The model under review builds one solid part; all positions refer to its coordinate system, in mm. Face numbers are marked on the shaded views. A direction names the side the tool comes from. Round coordinates to 2 decimals unless told otherwise and drop trailing zeros. Write each loop counter-clockwise with the first axis right and the second up, starting at its lowest first coordinate (ties: lowest second). Pieces come first, ordered by that corner, then holes. Notation, with made-up numbers: (-16.5, 72) -> (9.5, 72) arc R22 ccw to (9.5, 109) -> close; hole circle Ø9 at (-32.5, -24.75). An arc over 180 degrees is marked (long way). Answer in a Markdown table with one row per item. Add a question column.
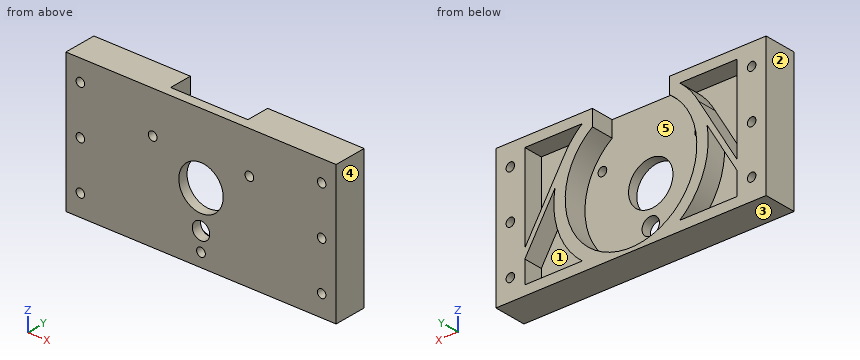
```python
from build123d import *

# Parameters (mm, degrees)
SKETCH1_W           = 140
SKETCH1_H           = 72
BOSS_EXTRUDE1_DEPTH = 17
SKETCH2_R           = 34.1
CUT_EXTRUDE1_DEPTH  = 12
SKETCH3_W           = 40
SKETCH3_H           = 24
CUT_EXTRUDE2_DEPTH  = 10
SKETCH4_R           = 2.2
CUT_EXTRUDE3_DEPTH  = 81.529497701
SKETCH5_R           = 2.25
SKETCH5_R_2         = 4.5
CUT_EXTRUDE4_DEPTH  = 80.62411695
CUT_EXTRUDE5_DEPTH  = 10
SKETCH7_R           = 11.5
CUT_EXTRUDE6_DEPTH  = 10


with BuildPart() as part:
    # Sketch1 → Boss-Extrude1 (new body)
    with BuildSketch(Plane(origin=(0, 0, 0), x_dir=(1, 0, 0), z_dir=(0, 1, 0))):
        Rectangle(SKETCH1_W, SKETCH1_H)
    extrude(amount=BOSS_EXTRUDE1_DEPTH)

    # Sketch2 → Cut-Extrude1 (cut)
    with BuildSketch(Plane(origin=(0, 17, 0), x_dir=(1, 0, 0), z_dir=(0, 1, 0))):
        with Locations(Location((0, 0, 0), (0, 0, 270))):
            Circle(SKETCH2_R)
    extrude(amount=-CUT_EXTRUDE1_DEPTH, mode=Mode.SUBTRACT)

    # Sketch3 → Cut-Extrude2 (cut)
    with BuildSketch(Plane.XY.offset(36)):
        with Locations((0, 17)):
            Rectangle(SKETCH3_W, SKETCH3_H)
    extrude(amount=-CUT_EXTRUDE2_DEPTH, mode=Mode.SUBTRACT)

    # Sketch4 → Cut-Extrude3 (cut, through all)
    with BuildSketch(Plane(origin=(0, 17, 0), x_dir=(1, 0, 0), z_dir=(0, 1, 0))):
        with Locations(Location((-62.5, 25, 0), (0, 0, 270))):
            Circle(SKETCH4_R)
        with Locations(Location((-62.5, 0, 0), (0, 0, 270))):
            Circle(SKETCH4_R)
        with Locations(Location((-62.5, -25, 0), (0, 0, 270))):
            Circle(SKETCH4_R)
        with Locations(Location((62.5, -25, 0), (0, 0, 90))):
            Circle(SKETCH4_R)
        with Locations(Location((62.5, 0, 0), (0, 0, 90))):
            Circle(SKETCH4_R)
        with Locations(Location((62.5, 25, 0), (0, 0, 90))):
            Circle(SKETCH4_R)
    extrude(amount=-CUT_EXTRUDE3_DEPTH, mode=Mode.SUBTRACT)

    # Sketch5 → Cut-Extrude4 (cut, through all)
    with BuildSketch(Plane(origin=(0, 5, 0), x_dir=(1, 0, 0), z_dir=(0, 1, 0))):
        with Locations(Location((0, 29, 0), (0, 0, 270))):
            Circle(SKETCH5_R)
        with Locations(Location((25.042343364, -14.374611046, 0), (0, 0, 270))):
            Circle(SKETCH5_R)
        with Locations(Location((-25.042343364, -14.374611046, 0), (0, 0, 270))):
            Circle(SKETCH5_R)
        with Locations(Location((0, 19.333592636, 0), (0, 0, 270))):
            Circle(SKETCH5_R_2)
    extrude(amount=-CUT_EXTRUDE4_DEPTH, mode=Mode.SUBTRACT)

    # Sketch6 → Cut-Extrude5 (cut)
    with BuildSketch(Plane(origin=(0, 17, 0), x_dir=(1, 0, 0), z_dir=(0, 1, 0))):
        with BuildLine():
            Line((-55, 31), (-25.27844932, 31))
            ThreePointArc((-25.27844932, 31), (-37.491645865, 13.941896942), (-39.391334679, -6.951456838))
            Line((-39.391334679, -6.951456838), (-55, 19.35498509))
            Line((-55, 19.35498509), (-55, 31))
        make_face()
        with BuildLine():
            Line((-55, -31), (-25.27844932, -31))
            ThreePointArc((-25.27844932, -31), (-30.757821307, -25.5725718), (-35.093761786, -19.194475343))
            Line((-35.093761786, -19.194475343), (-55, 14.35498509))
            Line((-55, 14.35498509), (-55, -31))
        make_face()
        with BuildLine():
            Line((55, -31), (25.27844932, -31))
            ThreePointArc((25.27844932, -31), (30.757821307, -25.5725718), (35.093761786, -19.194475343))
            Line((35.093761786, -19.194475343), (55, 14.35498509))
            Line((55, 14.35498509), (55, -31))
        make_face()
        with BuildLine():
            Line((55, 31), (55, 19.35498509))
            Line((55, 19.35498509), (39.391334679, -6.951456838))
            ThreePointArc((39.391334679, -6.951456838), (37.491645865, 13.941896942), (25.27844932, 31))
            Line((25.27844932, 31), (55, 31))
        make_face()
    extrude(amount=-CUT_EXTRUDE5_DEPTH, mode=Mode.SUBTRACT)

    # Sketch7 → Cut-Extrude6 (cut)
    with BuildSketch(Plane(origin=(0, 5, 0), x_dir=(1, 0, 0), z_dir=(0, 1, 0))):
        with Locations(Location((0, 0, 0), (0, 0, 270))):
            Circle(SKETCH7_R)
    extrude(amount=-CUT_EXTRUDE6_DEPTH, mode=Mode.SUBTRACT)


solid = part.part
```
1. Add section C-C on z = 4.5. Write out the cut boundary in (x, y).
2. Insertion check: pin 1 Ø3.5 at (x, z) = (-25.04, 14.37) entering from -Y; pin 2 Ø1 at (x, z) = (-48, 21) entering from +Y; pin 3 Ø5 at (x, z) = (0, -29) entering from +Y. Each pin has a flat end and moves straight along its axis. Give the tip position at first contact, or say it passes through.
3. Add section A-A on x = 0. Write out the cut boundary in (y, z).
4. For L1, parallel to Z at x = 62.5, y = 10.25; L2, parallel to X at y = 1.5, z = 0; L3, parallel to X at y = 1.2, z = -29, list the stretches that pass through material, from the lowest coordinate up.
5. Add section B-B on y = 9.5. State how many separate pieces and enclosed holes the cut face has, plus the area to 3 significant figures.
6. Tool access review of the marked faces 4 and 5: name each direction out of +Z, -Z, +X, -X, +Y, -Y from which nothing blocks a thin tool from reaching the whole face with its end or side.
7. Mouldability with a two-part tool opening along X and no side actions: class the marked faces 1, 2 and 3 as pulls with the +X half, pulls with the -X half, needs draft (parallel to the pull), parting line crosses it, or undercut.
8. Add section D-D on x = -62.5. Write out the cut boundary in (y, z).
Filled in:
| question | item | result |
|---|---|---|
| 1 | outline | (-70, 0) -> (-10.58, 0) -> (-10.58, 5) -> (-33.8, 5) -> (-33.8, 17) -> (-39.75, 17) -> (-39.75, 7) -> (-40.85, 7) -> (-40.85, 17) -> (-43.81, 17) -> (-43.81, 7) -> (-55, 7) -> (-55, 17) -> (-70, 17) -> close; (10.58, 0) -> (70, 0) -> (70, 17) -> (55, 17) -> (55, 7) -> (43.81, 7) -> (43.81, 17) -> (40.85, 17) -> (40.85, 7) -> (39.75, 7) -> (39.75, 17) -> (33.8, 17) -> (33.8, 5) -> (10.58, 5) -> close |
| 2 | pin 1 | through |
| 2 | pin 2 | y = 7 |
| 2 | pin 3 | y = 5 |
| 3 | outline | (0, -36) -> (17, -36) -> (17, -34.1) -> (5, -34.1) -> (5, -31.25) -> (0, -31.25) -> close; (0, -26.75) -> (5, -26.75) -> (5, -23.83) -> (0, -23.83) -> close; (0, -14.83) -> (5, -14.83) -> (5, -11.5) -> (0, -11.5) -> close; (0, 11.5) -> (5, 11.5) -> (5, 36) -> (0, 36) -> close |
| 4 | L1 | -36 to -27.2, -22.8 to -2.2, 2.2 to 22.8, 27.2 to 36 |
| 4 | L2 | -70 to -64.7, -60.3 to -11.5, 11.5 to 60.3, 64.7 to 70 |
| 4 | L3 | -70 to -2.25, 2.25 to 70 |
| 5 | separate pieces | 1 |
| 5 | enclosed holes | 10 |
| 5 | area | 3,930 mm² |
| 6 | face 4 | +Z, -Z, +X, +Y, -Y |
| 6 | face 5 | +Y |
| 7 | face 1 | undercut |
| 7 | face 2 | pulls with the -X half |
| 7 | face 3 | needs draft |
| 8 | outline | (0, -36) -> (17, -36) -> (17, -27.2) -> (0, -27.2) -> close; (0, -22.8) -> (17, -22.8) -> (17, -2.2) -> (0, -2.2) -> close; (0, 2.2) -> (17, 2.2) -> (17, 22.8) -> (0, 22.8) -> close; (0, 27.2) -> (17, 27.2) -> (17, 36) -> (0, 36) -> close |
